Could you check a few things on this model? Use its own coordinates, in mm. Round coordinates to 2 decimals unless told otherwise and drop trailing zeros. Order: outer loops, then holes, each group sorted by start corner. A loop starts at its lowest first (then second) coordinate and runs counter-clockwise, first axis right, second up. Notation, with made-up numbers: (71.5, -31) -> (87.5, -31) arc R27 ccw to (87.5, -8) -> close; hole circle Ø5 at (-19.5, 47). An arc over 180 degrees is marked (long way). One line per question, with ' | ' between items.
```python
from build123d import *

# Parameters (mm, degrees)
SKETCH1_R           = 40
SKETCH1_R_2         = 1.5
BOSS_EXTRUDE1_DEPTH = 4
SKETCH2_R           = 2.5
BOSS_EXTRUDE2_DEPTH = 6
FILLET1_R           = 3


with BuildPart() as part:
    # Sketch1 → Boss-Extrude1 (new body)
    with BuildSketch(Plane(origin=(0, 0, 0), x_dir=(1, 0, 0), z_dir=(0, 1, 0))):
        with Locations(Location((0, 0, 0), (0, 0, 270))):
            Circle(SKETCH1_R)
        with Locations(Location((0, -12.5, 0), (0, 0, 270))):
            Circle(SKETCH1_R_2, mode=Mode.SUBTRACT)
        with Locations(Location((-12.5, 0, 0), (0, 0, 270))):
            Circle(SKETCH1_R_2, mode=Mode.SUBTRACT)
        with Locations(Location((0, 12.5, 0), (0, 0, 270))):
            Circle(SKETCH1_R_2, mode=Mode.SUBTRACT)
        with Locations(Location((12.5, 0, 0), (0, 0, 270))):
            Circle(SKETCH1_R_2, mode=Mode.SUBTRACT)
    extrude(amount=BOSS_EXTRUDE1_DEPTH)

    # Sketch2 → Boss-Extrude2 (add)
    with BuildSketch(Plane(origin=(0, 4, 0), x_dir=(1, 0, 0), z_dir=(0, 1, 0))):
        with Locations(Location((30.310889132, 17.5, 0), (0, 0, 270))):
            Circle(SKETCH2_R)
        with Locations(Location((-30.310889132, -17.5, 0), (0, 0, 270))):
            Circle(SKETCH2_R)
    extrude(amount=BOSS_EXTRUDE2_DEPTH)

    # Fillet1
    fillet1_edges = [part.edges().sort_by_distance(p)[0] for p in [
        (30.310889132, 4, -20),
        (-30.310889132, 4, 15),
    ]]
    fillet(fillet1_edges, radius=FILLET1_R)


solid = part.part
```
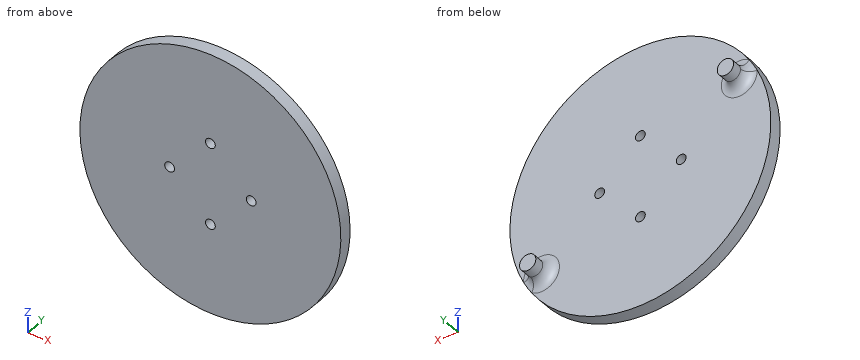
1. I want a section at A-A on z = 0. List the corners of the cut face in (x, y) for me, and give its area (3 significant figures).
From the geometry:
outline: (-40, 0) -> (-14, 0) -> (-14, 4) -> (-40, 4) -> close; (-11, 0) -> (11, 0) -> (11, 4) -> (-11, 4) -> close; (14, 0) -> (40, 0) -> (40, 4) -> (14, 4) -> close | area: 296 mm²
2. I want a section at B-B on x = 0. List the corners of the cut face in (y, z) for me.
From the geometry:
outline: (0, -40) -> (4, -40) -> (4, -14) -> (0, -14) -> close; (0, -11) -> (4, -11) -> (4, 11) -> (0, 11) -> close; (0, 14) -> (4, 14) -> (4, 40) -> (0, 40) -> close
3. I want a section at C-C on y = 1. List the corners of the cut face in (x, z) for me, and give its area (3 significant figures).
From the geometry:
outline: circle Ø80 at (0, 0); hole circle Ø3 at (-12.5, 0); hole circle Ø3 at (0, -12.5); hole circle Ø3 at (0, 12.5); hole circle Ø3 at (12.5, 0) | area: 5,000 mm²
4. I want a section at D-D on x = 12.5. List the corners of the cut face in (y, z) for me, and give its area (3 significant figures).
From the geometry:
outline: (0, -38) -> (4, -38) -> (4, -1.5) -> (0, -1.5) -> close; (0, 1.5) -> (4, 1.5) -> (4, 38) -> (0, 38) -> close | area: 292 mm²
5. I'm going to push flat-ended pins straight in: pin 1 (5 mm diameter, centred on y = 4.5, z = -6, fed in from +X); pin 2 (6 mm diameter, centred on x = -7.5, y = 3, fed in from +Z); pin 3 (3.5 mm diameter, centred on x = -12.5, z = 0, fed in from +Y). Where does each tip first touch, or does it pass through?
From the geometry:
pin 1: stops at x = 39.84 | pin 2: stops at z = 39.75 | pin 3: stops at y = 4
6. I need wall thicknesses on probe 1 along X at (y, z) = (2.15, 0); probe 2 along Y at (x, z) = (-23.5, -12); probe 3 along X at (y, z) = (6.5, 15.5). Which ranges of each line are inside material? Lowest first, please.
From the geometry:
probe 1: x = -40 to -14, -11 to 11, 14 to 40 | probe 2: y = 0 to 4 | probe 3: x = -31.88 to -28.74
